The listing builds one solid part. Answer for the finished solid, in the listing's coordinates (mm). Coordinates: 2 decimals unless noted, no trailing zeros. Order: outer loops, then holes, each group sorted by start corner. A loop starts at its lowest first (then second) coordinate and runs counter-clockwise, first axis right, second up. Notation, with made-up numbers: (10, -5.75) -> (22, -5.75) arc R20 ccw to (22, 33.25) -> close; hole circle Ø1 at (-3.75, 81.25). An arc over 180 degrees is marked (long way). One line per question, with ' | ' between items.
from build123d import *

# Parameters (mm, degrees)
SKETCH1_R           = 1.5
BOSS_EXTRUDE1_DEPTH = 1.6


with BuildPart() as part:
    # Sketch1 → Boss-Extrude1 (new body)
    with BuildSketch(Plane(origin=(0, 0, 0), x_dir=(1, 0, 0), z_dir=(0, 1, 0))):
        Polygon((46, -28.808269535), (35, -28.808269535), (35, -37.808269535), (-46, -37.808269535), (-46, 42.191730465), (46, 42.191730465), align=None)
        with Locations(Location((29.5, -35.308269535, 0), (0, 0, 270))):
            Circle(SKETCH1_R, mode=Mode.SUBTRACT)
        with Locations(Location((14, -35.308269535, 0), (0, 0, 270))):
            Circle(SKETCH1_R, mode=Mode.SUBTRACT)
        with Locations(Location((-31.5, -35.308269535, 0), (0, 0, 270))):
            Circle(SKETCH1_R, mode=Mode.SUBTRACT)
        with BuildLine():
            Line((-38, -36.808269535), (-42, -36.808269535))
            ThreePointArc((-42, -36.808269535), (-43.5, -35.308269535), (-42, -33.808269535))
            Line((-42, -33.808269535), (-38, -33.808269535))
            ThreePointArc((-38, -33.808269535), (-36.5, -35.308269535), (-38, -36.808269535))
        make_face(mode=Mode.SUBTRACT)
    extrude(amount=BOSS_EXTRUDE1_DEPTH)


solid = part.part
Item 1: Section B-B, the plane y = 0.7 is taken. Give the vertices of the cut face in (x, z), plus the area to 3 significant figures.
Computed values:
outline: (-46, -42.19) -> (46, -42.19) -> (46, 28.81) -> (35, 28.81) -> (35, 37.81) -> (-46, 37.81) -> close; hole (-42, 33.81) -> (-38, 33.81) arc R1.5 ccw to (-38, 36.81) -> (-42, 36.81) arc R1.5 ccw to start; hole circle Ø3 at (-31.5, 35.31); hole circle Ø3 at (14, 35.31); hole circle Ø3 at (29.5, 35.31) | area: 7,220 mm^2
Item 2: Find the intervals of material crossed by L1, parallel to Z at x = -38, y = 0.8; L2, parallel to Z at x = 30.5, y = 1.05; L3, parallel to X at y = 1.25, z = 31, in increasing order.
Computed values:
L1: z = -42.19 to 33.81, 36.81 to 37.81 | L2: z = -42.19 to 34.19, 36.43 to 37.81 | L3: x = -46 to 35
Item 3: Section A-A, the plane x = -31.5 is taken. Give the vertices of the cut face in (y, z), plus the area to 3 significant figures.
Computed values:
outline: (0, -42.19) -> (1.6, -42.19) -> (1.6, 33.81) -> (0, 33.81) -> close; (0, 36.81) -> (1.6, 36.81) -> (1.6, 37.81) -> (0, 37.81) -> close | area: 123 mm^2
Item 4: This flat-tipped pin is pushed along its axis until it touches: pin 1 Ø3.5 at (x, z) = (14, 35.31) entering from -Y. Where does it stop, or does it pass through?
Computed values:
pin 1: stops at y = 0
Item 5: Determine the mould class of faces 1 (the face through (-30.49, 0.79, 34.2)), 2 (the face through (1, 1.6, -3)), 3 (the face through (30.51, 0.79, 34.2)) for opening direction Z: pulls with the +Z half, pulls with the -Z half, needs draft (parallel to the pull), parting line crosses it, or undercut.
Computed values:
face 1: undercut | face 2: needs draft | face 3: undercut
